Read the model definition and answer for the solid it produces. Units are mm, in the model's axes. A direction names the side the tool comes from. Give positions to 0.01 mm unless a question says otherwise; leave off trailing zeros. Write each loop counter-clockwise with the first axis right and the second up, starting at its lowest first coordinate (ties: lowest second). Pieces come first, ordered by that corner, then holes.
```python
from build123d import *

# Parameters (mm, degrees)
SKETCH2_R                        = 33
CUT_EXTRUDE1_DEPTH               = 5.3
SKETCH3_R                        = 3.3
CUT_EXTRUDE2_DEPTH               = 178.522951756
M8X1_25_TAPPED_HOLE2_D           = 6.8
M8X1_25_TAPPED_HOLE2_DEPTH       = 23.75
M8X1_25_TAPPED_HOLE2_CSINK_D     = 8.05
M8X1_25_TAPPED_HOLE2_CSINK_ANGLE = 90
M8X1_25_TAPPED_HOLE2_TIP         = 2.042926105
M5X0_8_TAPPED_HOLE2_D            = 4.2
M5X0_8_TAPPED_HOLE2_CSINK_D      = 5.05
M5X0_8_TAPPED_HOLE2_CSINK_ANGLE  = 90


with BuildPart() as part:
    # Sketch1 → Revolve1 (revolve)
    with BuildSketch(Plane(origin=(0, 0, 0), x_dir=(0, 0, -1), z_dir=(1, 0, 0)), mode=Mode.PRIVATE) as revolve1_sk:
        Polygon((-17.35, 0), (-70, 0), (-70, 5.36), (-91, 5.36), (-91, 48.12), (-90.5, 48.12), (-90.5, 57.86), (-70, 57.86), (-70, 65.62), (-29.6, 65.62), (-29.6, 79.12), (-49.91, 79.12), (-49.91, 85.12), (-25, 85.12), (-25, 94.12), (-20, 94.12), (-20, 127.64), (-17.35, 127.64), align=None)
    revolve(revolve1_sk.sketch.rotate(Axis((0, -94.12, 0), (0, 1, 0)), 180), axis=Axis((0, -94.12, 0), (0, 1, 0)))

    # Sketch2 → Cut-Extrude1 (cut)
    with BuildSketch(Plane.XZ):
        with Locations(Location((0, 0, 0), (0, 0, 270))):
            Circle(SKETCH2_R)
    extrude(amount=-CUT_EXTRUDE1_DEPTH, mode=Mode.SUBTRACT)

    # Sketch3 → Cut-Extrude2 (cut, through all)
    with BuildSketch(Plane.XZ.offset(-5.36)):
        with Locations(Location((-84.5, 0, 0), (0, 0, 270))):
            Circle(SKETCH3_R)
        with Locations(Location((-73.17914662, 42.25, 0), (0, 0, 270))):
            Circle(SKETCH3_R)
        with Locations(Location((-42.25, 73.17914662, 0), (0, 0, 270))):
            Circle(SKETCH3_R)
        with Locations(Location((0, 84.5, 0), (0, 0, 270))):
            Circle(SKETCH3_R)
        with Locations(Location((42.25, 73.17914662, 0), (0, 0, 270))):
            Circle(SKETCH3_R)
        with Locations(Location((73.17914662, 42.25, 0), (0, 0, 270))):
            Circle(SKETCH3_R)
        with Locations(Location((84.5, 0, 0), (0, 0, 270))):
            Circle(SKETCH3_R)
        with Locations(Location((73.17914662, -42.25, 0), (0, 0, 270))):
            Circle(SKETCH3_R)
        with Locations(Location((42.25, -73.17914662, 0), (0, 0, 270))):
            Circle(SKETCH3_R)
        with Locations(Location((0, -84.5, 0), (0, 0, 270))):
            Circle(SKETCH3_R)
        with Locations(Location((-42.25, -73.17914662, 0), (0, 0, 270))):
            Circle(SKETCH3_R)
        with Locations(Location((-73.17914662, -42.25, 0), (0, 0, 270))):
            Circle(SKETCH3_R)
    extrude(amount=-CUT_EXTRUDE2_DEPTH, mode=Mode.SUBTRACT)

    # M8x1.25 Tapped Hole2
    with Locations(Plane(origin=(0, 0, 0), x_dir=(-1, 0, 0), z_dir=(0, -1, 0))):
        with Locations((15.011504616, 56.023697925), (-29, 50.229473419), (-56.023697925, 15.011504616), (-50.229473419, -29), (-15.011504616, -56.023697925), (29, -50.229473419), (56.023697925, -15.011504616), (50.229473419, 29)):
            CounterSinkHole(M8X1_25_TAPPED_HOLE2_D / 2, M8X1_25_TAPPED_HOLE2_CSINK_D / 2, depth=M8X1_25_TAPPED_HOLE2_DEPTH, counter_sink_angle=M8X1_25_TAPPED_HOLE2_CSINK_ANGLE)
            with Locations((0, 0, -(M8X1_25_TAPPED_HOLE2_DEPTH + M8X1_25_TAPPED_HOLE2_TIP / 2))):  # 118° drill point
                Cone(0, M8X1_25_TAPPED_HOLE2_D / 2, M8X1_25_TAPPED_HOLE2_TIP, mode=Mode.SUBTRACT)

    # M5x0.8 Tapped Hole2 (through all)
    with Locations(Plane(origin=(0, 57.86, 0), x_dir=(1, 0, 0), z_dir=(0, 1, 0))):
        with Locations((-21.870209311, 81.620732321), (21.870209311, -81.620732321)):
            CounterSinkHole(M5X0_8_TAPPED_HOLE2_D / 2, M5X0_8_TAPPED_HOLE2_CSINK_D / 2, counter_sink_angle=M5X0_8_TAPPED_HOLE2_CSINK_ANGLE)


solid = part.part
```
Item 1: Find the intervals of material crossed by line 1 along Y through (x, z) = (4, 30.5); line 2 along X through (y, z) = (30, 42); line 3 along Y through (x, z) = (27.5, -22), in increasing order.
Result set:
line 1: y = 5.3 to 65.62, 79.12 to 85.12
line 2: x = -80.73 to -76.47, -69.89 to 69.89, 76.47 to 80.73
line 3: y = 0 to 65.62, 79.12 to 85.12
Item 2: Section B-B (y = 20) is taken. Give the number of separate pieces and of enclosed holes in the cut face, and give its area (3 significant figures).
Result set:
separate pieces: 1
enclosed holes: 23
area: 24,300 mm2
Item 3: Determine the mould class of faces 3 (the cylindrical face through (0.1, 31.2, 87.8)), 4 (the cylindrical face through (-42.105, 31.243, 76.476)), 5 (the cylindrical face through (-42.084, 82.162, -26.831)), 6 (the flat face through (30, 65.62, 1)) for opening direction X: pulls with the +X half, pulls with the -X half, needs draft (parallel to the pull), parting line crosses it, or undercut.
Result set:
face 3: undercut
face 4: undercut
face 5: parting line crosses it
face 6: needs draft
Item 4: Which of the six approach directions +Z, -Z, +X, -X, +Y, -Y give full straight-line access (tool end or side, diameter ignored) to faces 1 (the cylindrical face through (87.77, 31.24, 0.43)), 2 (the cylindrical face through (30.828, 12.349, -53.096))?
Result set:
face 1: +Y, -Y
face 2: -Y
Item 5: Section C-C (z = -42.25) is taken. Write down the section's boundary in (x, y).
Result set:
outline: (-80.6, 5.36) - (-76.48, 5.36) - (-76.48, 57.86) - (-80.03, 57.86) - (-80.03, 48.12) - (-80.6, 48.12) - close; (-69.88, 5.36) - (-55.81, 5.36) - (-55.81, 0) - (55.81, 0) - (55.81, 5.36) - (69.88, 5.36) - (69.88, 57.86) - (55.81, 57.86) - (55.81, 65.62) - (-55.81, 65.62) - (-55.81, 57.86) - (-69.88, 57.86) - close; (-26.57, 79.12) - (26.57, 79.12) - (26.57, 85.12) - (-26.57, 85.12) - close; (76.48, 5.36) - (80.6, 5.36) - (80.6, 48.12) - (80.03, 48.12) - (80.03, 57.86) - (76.48, 57.86) - close
Item 6: Each of these flat-tipped pins is pushed along its axis until it touches: pin 1 Ø10 at (x, z) = (35, 44) entering from +Y; pin 2 Ø6 at (x, y) = (-16.5, 88) entering from +Z; pin 3 Ø8.5 at (x, z) = (73.18, 42.25) entering from +Y. Where does it stop, or does it pass through?
Result set:
pin 1: stops at y = 65.62
pin 2: stops at z = 47.39
pin 3: stops at y = 57.86
Item 7: Section A-A (x = -42.25) is taken. Write down the section's boundary in (y, z), and give its area (3 significant figures).
Result set:
outline: (0, -55.81) - (5.36, -55.81) - (5.36, -69.88) - (57.86, -69.88) - (57.86, -55.81) - (65.62, -55.81) - (65.62, 55.81) - (57.86, 55.81) - (57.86, 69.88) - (5.36, 69.88) - (5.36, 55.81) - (0, 55.81) - close; (5.36, -80.6) - (48.12, -80.6) - (48.12, -80.03) - (57.86, -80.03) - (57.86, -76.48) - (5.36, -76.48) - close; (5.36, 76.48) - (57.86, 76.48) - (57.86, 80.03) - (48.12, 80.03) - (48.12, 80.6) - (5.36, 80.6) - close; (79.12, -26.57) - (85.12, -26.57) - (85.12, 26.57) - (79.12, 26.57) - close
area: 9,540 mm2
Item 8: Section D-D (y = 71) is taken. Write down the section's boundary in (x, z).
Result set:
outline: circle Ø59.2 at (0, 0); hole circle Ø34.7 at (0, 0)
